The model under review builds one solid part; all positions refer to its coordinate system, in mm. A direction names the side the tool comes from. Give positions to 0.01 mm unless a question says otherwise; leave off trailing zeros. Loops run counter-clockwise (first coordinate to the right, second up) from the corner with the lowest first, then second, coordinate; pieces in that order, holes last. Notation, with made-up numbers: M 42,63 L 75,63 A28 ccw 75,81 Z; hole C 64,-19 d3. An arc over 180 degrees is marked long. Put each result on its own line as item: value. Start each with the question number.
```python
from build123d import *

# Parameters (mm, degrees)
F1_DEPTH = 20
F2_T     = -1
F3_R     = 24
F4_DEPTH = 19
F5_T     = -1
F7_DEPTH = 1


# Not quite as in the source:
# - a shell that OpenCascade refuses in one call is made with other operations: the cavity is built on its own and cut out


with BuildPart() as f1:
    # F0 (on Top) → F1 (new body)
    with BuildSketch(Plane.XY):
        Polygon((40, 50), (-40, 50), (-40, 40), (-50, 40), (-50, -40), (-40, -40), (-40, -50), (40, -50), (40, -40), (50, -40), (50, 40), (40, 40), align=None)
    extrude(amount=F1_DEPTH)

    # F2
    f2_openings = [f1.faces().sort_by_distance(p)[0] for p in [
        (0, 0, 20),
    ]]
    offset(amount=F2_T, openings=f2_openings, kind=Kind.INTERSECTION)

    # F3 (on face) → F4 (join)
    with BuildSketch(Plane.XY.offset(1)):
        Circle(F3_R)
    extrude(amount=F4_DEPTH)

    # F5: a shell. OpenCascade refuses it in one call, so the cavity is built on its own and cut out:
    # the body offset inwards by the wall thickness, plus a prism from it out through each open face.
    f5_core = offset(f1.part, amount=F5_T, kind=Kind.INTERSECTION, mode=Mode.PRIVATE)
    f5_exits = [f5_core.faces().sort_by_distance(p)[0] for p in [
        (0, 0, 19),
    ]]
    add(f5_core, mode=Mode.SUBTRACT)
    extrude(f5_exits, amount=-F5_T, mode=Mode.SUBTRACT)

    # F6 (on face) → F7 (join)
    with BuildSketch(Plane.XY.offset(20)):
        Polygon((-40, -50), (40, -50), (40, -40), (50, -40), (50, 40), (40, 40), (40, 50), (-40, 50), (-40, 40), (-50, 40), (-50, -40), (-40, -40), align=None)
    extrude(amount=F7_DEPTH)


solid = f1.part
```
Item 1: To check wall thickness, follow L1, parallel to Y at x = 0, z = 12.5; L2, parallel to Z at x = 16, y = 33.5; L3, parallel to X at y = -1.5, z = 17.75. State the ranges of each line that lie inside material, in increasing order. Write a range as [from, to].
Item 2: Consider section A-A, the plane z = 10.5. Write out the cut boundary in (x, y), plus the area to 3 significant figures.
Item 3: Draft analysis for pull direction Y (two halves, no side actions). For faces 1 (the flat face through (1, 49, 10)), 2 (the flat face through (-45, -40, 10)), 3 (the flat face through (-1, 1, 0)), state which applies: +Y half, -Y half, draft (parallel to the pull), parting line (faces both ways), or undercut.
Item 4: Consider section C-C, the plane y = 0. Write out the cut boundary in (x, z), plus the area to 3 significant figures.
Item 5: Tool access review of faces 4 (the flat face through (-40, -45, 10)), 5 (the flat face through (50, -1, 10)), 6 (the flat face through (40, 45, 10)), 7 (the flat face through (-1, 1, 21)), 8 (the flat face through (-44, -39, 10)): name each direction out of +Z, -Z, +X, -X, +Y, -Y from which nothing blocks a thin tool from reaching the whole face with its end or side.
Item 6: Clearance check with flat-ended pins moving along their axes: pin 1 Ø5 at (y, z) = (-44, 8) entering from +X; pin 2 Ø11 at (x, z) = (47, 8.5) entering from +Y; pin 3 Ø3 at (x, z) = (45, 13) entering from -Y; pin 4 Ø11 at (y, z) = (43, 11.5) entering from -X. State where each tip first meets the part, or that it passes through.
Item 7: Consider section B-B, the plane x = -41.5. Write out the cut boundary in (y, z), plus the area to 3 significant figures.
Report:
1. L1: [-50, -49], [-24, -23], [23, 24], [49, 50]
1. L2: [0, 1], [20, 21]
1. L3: [-50, -49], [-23.95, -22.95], [22.95, 23.95], [49, 50]
2. outline: M -50,-40 L -40,-40 L -40,-50 L 40,-50 L 40,-40 L 50,-40 L 50,40 L 40,40 L 40,50 L -40,50 L -40,40 L -50,40 Z; C 0,0 d48; hole M -49,-39 L -39,-39 L -39,-49 L 39,-49 L 39,-39 L 49,-39 L 49,39 L 39,39 L 39,49 L -39,49 L -39,39 L -49,39 Z; hole C 0,0 d46
2. area: 544 mm²
3. face 1: undercut
3. face 2: -Y half
3. face 3: draft
4. outline: M -50,0 L 50,0 L 50,21 L -50,21 Z; hole M -49,1 L -24,1 L -24,20 L -49,20 Z; hole M -23,1 L 23,1 L 23,20 L -23,20 Z; hole M 24,1 L 49,1 L 49,20 L 24,20 Z
4. area: 276 mm²
5. face 4: +Z, -Z, -X, -Y
5. face 5: +Z, -Z, +X, +Y, -Y
5. face 6: +Z, -Z, +X, +Y
5. face 7: +Z, +X, -X, +Y, -Y
5. face 8: none
6. pin 1: x = 40
6. pin 2: y = 40
6. pin 3: y = -40
6. pin 4: x = -50
7. outline: M -40,0 L 40,0 L 40,21 L -40,21 Z; hole M -39,1 L 39,1 L 39,20 L -39,20 Z
7. area: 198 mm²
